from build123d import *

# Parameters (mm, degrees)
FILLET1_R = 0.25


with BuildPart() as part:
    # Sketch1 → Revolve1 (revolve)
    with BuildSketch(Plane.XY):
        with BuildLine():
            Line((13.5, 8.080985965), (13.5, 0))
            Line((13.5, 0), (12.5, 0))
            Line((12.5, 0), (12.5, 8.080985965))
            ThreePointArc((12.5, 8.080985965), (12.177697445, 9.030458674), (11.343995274, 9.587520655))
            ThreePointArc((11.343995274, 9.587520655), (5.720941081, 10.706015676), (0, 11.080985965))
            Line((0, 11.080985965), (0, 12.080985965))
            ThreePointArc((0, 12.080985965), (5.851467273, 11.697460538), (11.60281432, 10.553446481))
            ThreePointArc((11.60281432, 10.553446481), (12.971050786, 9.639220103), (13.5, 8.080985965))
        make_face()
    revolve(axis=Axis((0, -281.832551031, 0), (0, 1, 0)))

    # Fillet1
    fillet1_edges = [part.edges().sort_by_distance(p)[0] for p in [
        (-13.5, 0, 0),
        (-12.5, 0, 0),
    ]]
    fillet(fillet1_edges, radius=FILLET1_R)


solid = part.part
CAD build for the part. Positions are in the model's coordinates, mm. Coordinates: 2 decimals unless noted, no trailing zeros. Loops run counter-clockwise (first coordinate to the right, second up) from the corner with the lowest first, then second, coordinate; pieces in that order, holes last. Notation, with made-up numbers: (26, 40.25) - (31, 40.25) arc R16 ccw to (31, 44.25) - close; hole circle Ø8 at (1.25, 22.25). An arc over 180 degrees is marked (long way). Write item = value, one per line. Start each with the question number.
Q1. Pull direction Z, two halves, no side cores. Call faces 1 (the cylindrical face through (-2.93, 4.11, 13.18)), 2 (the flat face through (-7, 0, -11)), 3 (the cylindrical face through (11.923, 4.22, -3.755)): pulls with the +Z half, pulls with the -Z half, needs draft (parallel to the pull), parting line crosses it, or undercut.
Q2. Drill centre lines: L1, parallel to Z at x = 0, y = 5; L2, parallel to Z at x = 2.5, y = 1.25. Where is each one in solid material? Low to high.
Q3. Flat gauge pins, fed straight in: pin 1 Ø2 at (y, z) = (7.5, 7) entering from +X; pin 2 Ø4 at (x, y) = (-6, 10.5) entering from -Z; pin 3 Ø4 at (y, z) = (10.5, 10.5) entering from +X; pin 4 Ø1 at (x, y) = (-0.5, 4.5) entering from +Z. Where does each tip first touch, or does it go through?
Q4. Cut at D-D, the plane y = 8.5. List the corners of the cut face in (x, z), then the cut area to 3 significant figures.
Q5. Cut at B-B, the plane z = 0. List the corners of the cut face in (x, y).
Q6. Cut at A-A, the plane x = 0. List the corners of the cut face in (y, z), then the cut area to 3 significant figures.
Q7. Cut at C-C, the plane y = 1. List the corners of the cut face in (x, z), then the cut area to 3 significant figures.
Computed:
q1.face_1 = parting line crosses it
q1.face_2 = needs draft
q1.face_3 = undercut
q2.L1 = -13.5 to -12.5, 12.5 to 13.5
q2.L2 = -13.27 to -12.25, 12.25 to 13.27
q3.pin_1 = 12.09
q3.pin_2 = -12.48
q3.pin_3 = 9.74
q3.pin_4 = 13.5
q4.outline = circle Ø26.93 at (0, 0); hole circle Ø24.89 at (0, 0)
q4.area = 83.2 mm²
q5.outline = (-13.5, 0.25) arc R0.25 ccw to (-13.25, 0) - (-12.75, 0) arc R0.25 ccw to (-12.5, 0.25) - (-12.5, 8.08) arc R1.56 cw to (-11.34, 9.59) arc R43.83 cw to (11.34, 9.59) arc R1.56 cw to (12.5, 8.08) - (12.5, 0.25) arc R0.25 ccw to (12.75, 0) - (13.25, 0) arc R0.25 ccw to (13.5, 0.25) - (13.5, 8.08) arc R2.56 ccw to (11.6, 10.55) arc R44.83 ccw to (-11.6, 10.55) arc R2.56 ccw to (-13.5, 8.08) - close
q6.outline = (0, -13.25) arc R0.25 ccw to (0.25, -13.5) - (8.08, -13.5) arc R2.56 ccw to (10.55, -11.6) arc R44.83 ccw to (10.55, 11.6) arc R2.56 ccw to (8.08, 13.5) - (0.25, 13.5) arc R0.25 ccw to (0, 13.25) - (0, 12.75) arc R0.25 ccw to (0.25, 12.5) - (8.08, 12.5) arc R1.56 cw to (9.59, 11.34) arc R43.83 cw to (9.59, -11.34) arc R1.56 cw to (8.08, -12.5) - (0.25, -12.5) arc R0.25 ccw to (0, -12.75) - close
q6.area = 44.7 mm²
q7.outline = circle Ø27 at (0, 0); hole circle Ø25 at (0, 0)
q7.area = 81.7 mm²
